Design review of the part built by this model. Coordinates are the model's own, in mm. A direction names the side the tool comes from. Round coordinates to 2 decimals unless told otherwise and drop trailing zeros. Write each loop counter-clockwise with the first axis right and the second up, starting at its lowest first coordinate (ties: lowest second). Pieces come first, ordered by that corner, then holes. Notation, with made-up numbers: (33.25, 55) - (58.25, 55) arc R20 cw to (58.25, 79) - close; hole circle Ø6 at (73.25, -25.75). An arc over 180 degrees is marked (long way). Use one line per item in the form item = value.
```python
from build123d import *

# Parameters (mm, degrees)
F1_DEPTH = 19.304
F3_DEPTH = 19.304
F4_R     = 11.1125
F5_DEPTH = 19.304
F6_W     = 19.304
F6_H     = 19.304
F7_DEPTH = 19.304


with BuildPart() as f1:
    # F0 (on Front) → F1 (new body)
    with BuildSketch(Plane.XZ):
        with BuildLine():
            Line((-67.056, 0), (0, 0))
            Line((0, 0), (0, 53.34))
            ThreePointArc((0, 53.34), (-33.528, 86.868), (-67.056, 53.34))
            Line((-67.056, 53.34), (-67.056, 0))
        make_face()
    extrude(amount=F1_DEPTH)

    # F0 (on Front) → F3 (join)
    with BuildSketch(Plane.XZ):
        with BuildLine():
            Line((-67.056, 0), (0, 0))
            Line((0, 0), (0, 53.34))
            ThreePointArc((0, 53.34), (-33.528, 86.868), (-67.056, 53.34))
            Line((-67.056, 53.34), (-67.056, 0))
        make_face()
    extrude(amount=F3_DEPTH)

    # F4 (on face) → F5 (cut)
    with BuildSketch(Plane.XZ.offset(19.304)):
        with Locations((-33.439703, 64.4525)):
            Circle(F4_R)
    extrude(amount=-F5_DEPTH, mode=Mode.SUBTRACT)

    # F6 (on face) → F7 (join)
    with BuildSketch(Plane.XZ.offset(19.304)):
        with Locations((-9.652, 9.652)):
            Rectangle(F6_W, F6_H)
    extrude(amount=F7_DEPTH)


solid = f1.part
```
Q1. We need section B-B on x = -28. Write out the cut boundary in (y, z), then the cut area to 3 significant figures.
Calculated:
outline = (-19.3, 0) - (0, 0) - (0, 54.76) - (-19.3, 54.76) - close; (-19.3, 74.14) - (0, 74.14) - (0, 86.41) - (-19.3, 86.41) - close
area = 1,290 mm2
Q2. Machinability: for faces 4 (the flat face through (-19.304, -29, 10)), 5 (the flat face through (-10, -29, 19.304)), 6 (the flat face through (-10, -38.608, 10)), which of the approach directions +Z, -Z, +X, -X, +Y, -Y give a long, thin tool a straight path to every point of the face, cutting with its end or side? Answer none if there is none.
Calculated:
face_4 = +Z, -Z, -X, -Y
face_5 = +Z, +X, -X, -Y
face_6 = +Z, -Z, +X, -X, -Y
Q3. Draft analysis for pull direction Z (two halves, no side actions). For faces 1 (the flat face through (0, -15, 20)), 2 (the flat face through (-27, -15, 0)), 3 (the cylindrical face through (-27.466, -9.787, 73.823)), state which applies: released by +Z, released by -Z, zero draft, split by the parting line, or undercut.
Calculated:
face_1 = zero draft
face_2 = released by -Z
face_3 = undercut
Q4. We need section C-C on z = 13.5. Write out the cut boundary in (x, y).
Calculated:
outline = (-67.06, -19.3) - (-19.3, -19.3) - (-19.3, -38.61) - (0, -38.61) - (0, 0) - (-67.06, 0) - close
Q5. For P1, Ø5, axis at y = -10.5, z = 61, coming from the -X side; P2, Ø12, axis at x = -37, y = -28, coming from the -Z side; P3, Ø9.5, axis at x = -12.5, y = -30, coming from the +Z side; P4, Ø4, axis at x = -55, z = 51.5, coming from the -Y side, all flat-tipped, find the tip position at first contact; note any pin that passes through.
Calculated:
P1 = -66.66
P2 = through
P3 = 19.3
P4 = -19.3
Q6. We need section D-D on y = -7. Write out the cut boundary in (x, z) (1 decimal).
Calculated:
outline = (-67.1, 0) - (0, 0) - (0, 53.3) arc R33.5 ccw to (-67.1, 53.3) - close; hole circle Ø22.2 at (-33.4, 64.5)
Q7. We need section A-A on z = 74.5. Write out the cut boundary in (x, y), then the cut area to 3 significant figures.
Calculated:
outline = (-59.54, -19.3) - (-38.19, -19.3) - (-38.19, 0) - (-59.54, 0) - close; (-28.69, -19.3) - (-7.52, -19.3) - (-7.52, 0) - (-28.69, 0) - close
area = 821 mm2
Q8. To check wall thickness, follow line 1 along Y through (x, z) = (-57, 68); line 2 along Z through (x, y) = (-23.5, -7.5); line 3 along X through (y, z) = (-11.5, 62). State the ranges of each line that lie inside material, in increasing order. Write a range as from..to.
Calculated:
line_1 = -19.3..0
line_2 = 0..59.48, 69.42..85.33
line_3 = -65.92..-44.28, -22.6..-1.14
